The listing builds one solid part. Answer for the finished solid, in the listing's coordinates (mm). Face numbers are marked on the shaded views. Round coordinates to 2 decimals unless told otherwise and drop trailing zeros. Write each loop counter-clockwise with the first axis right and the second up, starting at its lowest first coordinate (ties: lowest second). Pieces come first, ordered by that corner, then holes. Notation, with made-up numbers: (-29, 73) - (25, 73) arc R27 ccw to (25, 90) - close; hole circle Ø10 at (21, 68.25). An arc over 180 degrees is marked (long way). Answer as CSV lines item,"result". Start each with the question number.
Item 1: A cutting plane is placed at C-C on x = 13. Determine the outline of the cut face in (y, z), and give its area (3 significant figures).
Item 2: Straight lines are drawn through the part: line 1 along Z through (x, y) = (12, 0.4); line 2 along X through (y, z) = (2.55, -8.6); line 3 along X through (y, z) = (0.35, -20). For each, find the intervals that lie inside material, in ascending order. Write a range as [from, to].
Item 3: For a pull along Z with two mould halves and no side action, classify the marked faces 1, 2 and 3 as pulls with the +Z half, pulls with the -Z half, needs draft (parallel to the pull), parting line crosses it, or undercut.
Item 4: A cutting plane is placed at B-B on y = 2.3. Determine the outline of the cut face in (x, z), and give its area (3 significant figures).
Item 5: Flat-ended cylindrical pins translate along their axes: pin 1 (1 mm diameter, centred on y = 1.5, z = -21, fed in from -X); pin 2 (4.5 mm diameter, centred on x = 11.8, z = -21.4, fed in from -Y). Find the tip coordinate at first contact, or state that the pin passes through.
Item 6: A cutting plane is placed at D-D on y = 0.7. Determine the outline of the cut face in (x, z).
Item 7: A cutting plane is placed at A-A on z = -21.4. Determine the outline of the cut face in (x, y), and give its area (3 significant figures).
```python
from build123d import *

# Parameters (mm, degrees)
SKETCH_1_W          = 15.8
SKETCH_1_H          = 30
EXTRUDE_1_DEPTH     = 4
SKETCH_2_R          = 2.05
CUT_EXTRUDE_1_DEPTH = 35.141470384
CUT_EXTRUDE_2_DEPTH = 2


with BuildPart() as part:
    # Sketch 1 → Extrude 1 (new body)
    with BuildSketch(Plane(origin=(0, 0, 0), x_dir=(1, 0, 0), z_dir=(0, 1, 0))):
        with Locations((7.9, 15)):
            Rectangle(SKETCH_1_W, SKETCH_1_H)
    extrude(amount=EXTRUDE_1_DEPTH)

    # Sketch 2 → Cut-Extrude 1 (cut, through all)
    with BuildSketch(Plane(origin=(0, 4, 0), x_dir=(1, 0, 0), z_dir=(0, 1, 0))):
        with Locations(Location((11.8, 21.4, 0), (0, 0, 270))):
            Circle(SKETCH_2_R)
        with Locations(Location((11.8, 8.6, 0), (0, 0, 270))):
            Circle(SKETCH_2_R)
    extrude(amount=-CUT_EXTRUDE_1_DEPTH, mode=Mode.SUBTRACT)

    # Sketch 5 → Cut-Extrude 2 (cut)
    with BuildSketch(Plane.XZ):
        Polygon((14.55, -7.01228676), (11.8, -5.424573519), (9.05, -7.01228676), (9.05, -10.18771324), (11.8, -11.775426481), (14.55, -10.18771324), align=None)
        Polygon((9.05, -22.98771324), (11.8, -24.575426481), (14.55, -22.98771324), (14.55, -19.81228676), (11.8, -18.224573519), (9.05, -19.81228676), align=None)
    extrude(amount=-CUT_EXTRUDE_2_DEPTH, mode=Mode.SUBTRACT)


solid = part.part
```
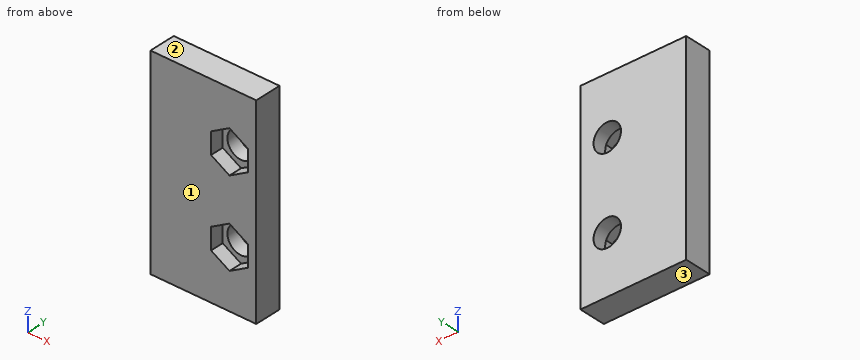
Geometry says:
1,outline,"(0, -30) - (4, -30) - (4, -23.06) - (2, -23.06) - (2, -23.88) - (0, -23.88) - close; (0, -18.92) - (2, -18.92) - (2, -19.74) - (4, -19.74) - (4, -10.26) - (2, -10.26) - (2, -11.08) - (0, -11.08) - close; (0, -6.12) - (2, -6.12) - (2, -6.94) - (4, -6.94) - (4, 0) - (0, 0) - close"
1,area,"86.8 mm^2"
2,line 1,"z = [-30, -24.46], [-18.34, -11.66], [-5.54, 0]"
2,line 2,"x = [0, 9.75], [13.85, 15.8]"
2,line 3,"x = [0, 9.05], [14.55, 15.8]"
3,face 1,"needs draft"
3,face 2,"pulls with the +Z half"
3,face 3,"pulls with the -Z half"
4,outline,"(0, -30) - (15.8, -30) - (15.8, 0) - (0, 0) - close; hole circle Ø4.1 at (11.8, -21.4); hole circle Ø4.1 at (11.8, -8.6)"
4,area,"448 mm^2"
5,pin 1,"stops at x = 0"
5,pin 2,"stops at y = 2"
6,outline,"(0, -30) - (15.8, -30) - (15.8, 0) - (0, 0) - close; hole (9.05, -22.99) - (11.8, -24.58) - (14.55, -22.99) - (14.55, -19.81) - (11.8, -18.22) - (9.05, -19.81) - close; hole (9.05, -10.19) - (11.8, -11.78) - (14.55, -10.19) - (14.55, -7.01) - (11.8, -5.42) - (9.05, -7.01) - close"
7,outline,"(0, 0) - (9.05, 0) - (9.05, 2) - (9.75, 2) - (9.75, 4) - (0, 4) - close; (13.85, 2) - (14.55, 2) - (14.55, 0) - (15.8, 0) - (15.8, 4) - (13.85, 4) - close"
7,area,"44.0 mm^2"
